Design review of the part built by this model. Coordinates are the model's own, in mm. A direction names the side the tool comes from. Give positions to 0.01 mm unless a question says otherwise; leave off trailing zeros. Loops run counter-clockwise (first coordinate to the right, second up) from the corner with the lowest first, then second, coordinate; pieces in that order, holes last. Notation, with made-up numbers: (-27, 23) -> (7, 23) arc R21 cw to (7, 52) -> close; hole circle Ø1 at (46.25, 37). An arc over 180 degrees is marked (long way). Use a Markdown table: item, result. Add a question column.
1. Draft analysis for pull direction Z (two halves, no side actions). For faces 1 (the flat face through (0, 19, -5)), 2 (the flat face through (5, 19, -10)), 3 (the flat face through (6.5, 19, -3)), state which applies: pulls with the +Z half, pulls with the -Z half, needs draft (parallel to the pull), parting line crosses it, or undercut.
2. For faces 4 (the flat face through (6, 36, -4.5)), 5 (the flat face through (10, 19, -5)), 6 (the flat face through (5, 40, -5)), 7 (the flat face through (8, 0, -3)), 8 (the flat face through (3, 19, -6.5)), list the 3-axis set-ups (+Z, -Z, +X, -X, +Y, -Y) from which the entire face can be reached by the end or side of a thin tool; tool diameter is ignored.
3. To check wall thickness, follow line 1 (Y direction, x = 6.25, z = -9.5); line 2 (X direction, y = 26, z = -8.75); line 3 (Y direction, x = 9, z = -3.5). State the ranges of each line that lie inside material, in increasing order.
4. Add section D-D (x = 9). State the section outline as (y, z) points, and give its area (3 significant figures).
5. Add section A-A (z = -4). State the section outline as (x, y) points, and give its area (3 significant figures).
6. Add section C-C (x = 5.75). State the section outline as (y, z) points, and give its area (3 significant figures).
7. For pin 1 Ø1.6 at (y, z) = (22, -3.5) entering from +X; pin 2 Ø1 at (x, y) = (6, 37) entering from -Z, all flat-tipped, find the tip position at first contact; note any pin that passes through.
8. Add section B-B (y = 11.5). State the section outline as (x, z) points, and give its area (3 significant figures).
```python
from build123d import *

# Parameters (mm, degrees)
SKETCH1_W           = 10
SKETCH1_H           = 10
BOSS_EXTRUDE1_DEPTH = 40
SKETCH3_W           = 7.5
SKETCH3_H           = 4
CUT_EXTRUDE1_DEPTH  = 7.5
SKETCH4_W           = 2
SKETCH4_H           = 5.5
CUT_EXTRUDE2_DEPTH  = 38
SKETCH5_W           = 10
SKETCH5_H           = 10
BOSS_EXTRUDE2_DEPTH = 2.5
BOSS_EXTRUDE3_REACH = 44.426
SKETCH6_W           = 1
SKETCH6_H           = 2


with BuildPart() as part:
    # Sketch1 → Boss-Extrude1 (new body)
    with BuildSketch(Plane(origin=(0, 0, 0), x_dir=(1, 0, 0), z_dir=(0, 1, 0))):
        with Locations((5, 5)):
            Rectangle(SKETCH1_W, SKETCH1_H)
    extrude(amount=BOSS_EXTRUDE1_DEPTH)

    # Sketch3 → Cut-Extrude1 (cut)
    with BuildSketch(Plane(origin=(0, 0, -10), x_dir=(-1, 0, 0), z_dir=(0, 0, -1))):
        with Locations((-6.25, 36)):
            Rectangle(SKETCH3_W, SKETCH3_H)
    extrude(amount=-CUT_EXTRUDE1_DEPTH, mode=Mode.SUBTRACT)

    # Sketch4 → Cut-Extrude2 (cut)
    with BuildSketch(Plane.XZ):
        Polygon((10, -2.5), (2.5, -2.5), (2.5, -4.5), (4.5, -4.5), (10, -4.5), align=None)
        with Locations((3.5, -7.25)):
            Rectangle(SKETCH4_W, SKETCH4_H)
    extrude(amount=-CUT_EXTRUDE2_DEPTH, mode=Mode.SUBTRACT)


with BuildPart() as cut_extrude2_piece_1:
    # of the separate pieces the step leaves, piece 1, a body of its own (cut_extrude2_pieces)
    add(part.part.solids().sort_by_distance((0, 0, 0))[0])



with BuildPart() as cut_extrude2_piece_2:
    # of the separate pieces the step leaves, piece 2, a body of its own (cut_extrude2_pieces)
    add(part.part.solids().sort_by_distance((10, 0, -4.5))[0])


with BuildPart() as cut_extrude2_piece_1_1:
    add(cut_extrude2_piece_1.part)

    add(cut_extrude2_piece_2.part)  # Boss-Extrude2 merges Cut-Extrude2 piece 2
    # Sketch5 → Boss-Extrude2 (add)
    with BuildSketch(Plane.XZ):
        with Locations((5, -5)):
            Rectangle(SKETCH5_W, SKETCH5_H)
    extrude(amount=BOSS_EXTRUDE2_DEPTH)

    # Boss-Extrude3: up to this face of the body (flat: up to its plane)
    boss_extrude3_end = Plane(cut_extrude2_piece_1_1.part.faces().sort_by_distance((6.25, 38, -6.25))[0])
    # Sketch6 → Boss-Extrude3 (add, up to the picked face)
    with BuildSketch(Plane(origin=(0, 0, 0), x_dir=(1, 0, 0), z_dir=(0, 1, 0)), mode=Mode.PRIVATE) as boss_extrude3_sk1:
        Polygon((3.5, 4.5), (3.5, 2.5), (6.5, 2.5), (6.5, 4.5), (4.5, 4.5), align=None)
    boss_extrude3_tool1 = split(extrude(boss_extrude3_sk1.sketch, amount=BOSS_EXTRUDE3_REACH, mode=Mode.PRIVATE), bisect_by=boss_extrude3_end, keep=Keep.BOTH, mode=Mode.PRIVATE)
    # Sketch6 → Boss-Extrude3 (add, up to the picked face)
    with BuildSketch(Plane(origin=(0, 0, 0), x_dir=(1, 0, 0), z_dir=(0, 1, 0)), mode=Mode.PRIVATE) as boss_extrude3_sk2:
        with Locations((4, 5.5)):
            Rectangle(SKETCH6_W, SKETCH6_H)
    boss_extrude3_tool2 = split(extrude(boss_extrude3_sk2.sketch, amount=BOSS_EXTRUDE3_REACH, mode=Mode.PRIVATE), bisect_by=boss_extrude3_end, keep=Keep.BOTH, mode=Mode.PRIVATE)
    # Sketch6 → Boss-Extrude3 (add, up to the picked face)
    with BuildSketch(Plane(origin=(0, 0, 0), x_dir=(1, 0, 0), z_dir=(0, 1, 0)), mode=Mode.PRIVATE) as boss_extrude3_sk3:
        with Locations((3, 5.5)):
            Rectangle(SKETCH6_W, SKETCH6_H)
    boss_extrude3_tool3 = split(extrude(boss_extrude3_sk3.sketch, amount=BOSS_EXTRUDE3_REACH, mode=Mode.PRIVATE), bisect_by=boss_extrude3_end, keep=Keep.BOTH, mode=Mode.PRIVATE)
    # Sketch6 → Boss-Extrude3 (add, up to the picked face)
    with BuildSketch(Plane(origin=(0, 0, 0), x_dir=(1, 0, 0), z_dir=(0, 1, 0)), mode=Mode.PRIVATE) as boss_extrude3_sk4:
        with Locations((3, 3.5)):
            Rectangle(SKETCH6_W, SKETCH6_H)
    boss_extrude3_tool4 = split(extrude(boss_extrude3_sk4.sketch, amount=BOSS_EXTRUDE3_REACH, mode=Mode.PRIVATE), bisect_by=boss_extrude3_end, keep=Keep.BOTH, mode=Mode.PRIVATE)
    add(boss_extrude3_tool1.solids().sort_by(Axis((5, 0, -3.5), (0, 1, 0)))[0])
    add(boss_extrude3_tool2.solids().sort_by(Axis((4, 0, -5.5), (0, 1, 0)))[0])
    add(boss_extrude3_tool3.solids().sort_by(Axis((3, 0, -5.5), (0, 1, 0)))[0])
    add(boss_extrude3_tool4.solids().sort_by(Axis((3, 0, -3.5), (0, 1, 0)))[0])


solid = cut_extrude2_piece_1_1.part
```
Taken from the geometry:
| question | item | result |
|---|---|---|
| 1 | face 1 | needs draft |
| 1 | face 2 | pulls with the -Z half |
| 1 | face 3 | undercut |
| 2 | face 4 | -Z, +X |
| 2 | face 5 | +Z, -Z, +X, +Y, -Y |
| 2 | face 6 | +Z, -Z, +X, -X, +Y |
| 2 | face 7 | +X |
| 2 | face 8 | -Z |
| 3 | line 1 | y = -2.5 to 34, 38 to 40 |
| 3 | line 2 | x = 0 to 2.5, 4.5 to 10 |
| 3 | line 3 | y = -2.5 to 0, 38 to 40 |
| 4 | outline | (-2.5, -10) -> (34, -10) -> (34, -4.5) -> (0, -4.5) -> (0, -2.5) -> (38, -2.5) -> (38, -10) -> (40, -10) -> (40, 0) -> (-2.5, 0) -> close |
| 4 | area | 327 mm^2 |
| 5 | outline | (0, -2.5) -> (10, -2.5) -> (10, 0) -> (6.5, 0) -> (6.5, 38) -> (10, 38) -> (10, 40) -> (0, 40) -> close |
| 5 | area | 292 mm^2 |
| 6 | outline | (-2.5, -10) -> (34, -10) -> (34, -4.5) -> (38, -4.5) -> (38, -10) -> (40, -10) -> (40, 0) -> (-2.5, 0) -> close |
| 6 | area | 403 mm^2 |
| 7 | pin 1 | stops at x = 6.5 |
| 7 | pin 2 | stops at z = -4.5 |
| 8 | outline | (0, -10) -> (2.5, -10) -> (2.5, -6.5) -> (4.5, -6.5) -> (4.5, -10) -> (10, -10) -> (10, -4.5) -> (6.5, -4.5) -> (6.5, -2.5) -> (10, -2.5) -> (10, 0) -> (0, 0) -> close |
| 8 | area | 86.0 mm^2 |
